Input: part model. Units: mm. Frame: model coordinates. Face numbers are marked on the shaded views. A direction names the side the tool comes from. Coordinates: 2 decimals unless noted, no trailing zeros. Loops run counter-clockwise (first coordinate to the right, second up) from the corner with the lowest first, then second, coordinate; pieces in that order, holes last. Notation, with made-up numbers: (9, -18.75) - (17, -18.75) arc R29 ccw to (17, 19.25) - close; hole circle Ø2 at (58.5, 2). An arc over 180 degrees is marked (long way). Use one line per item in the form item = value.
Autodesk Fusion 360 part; units mm, degrees
sketch "Back plate disc" plane through (0, 0, 0) normal (0, 0, 1) x (1, 0, 0)
  circle A0 centre (0, 0) radius 49
  dimension "d21" = 98
extrude "Main body extrude" add sketch "Back plate disc" along normal blind 23.2
sketch "Motor top outer ring sketch" plane through (0, 0, 23.2) normal (0, 0, 1) x (-1, 0, 0)
  circle A0 centre (0, 0) radius 49
  circle A1 centre (0, 0) radius 24
  dimension "d24" = 48
extrude "Motor top, outer ring extrude" add sketch "Motor top outer ring sketch" along normal blind 1.3 contours A1
sketch "Motor rotor ring sketch" plane through (0, 0, 24.5) normal (0, 0, 1) x (-1, 0, 0)
  circle A0 centre (0, 0) radius 24
  circle A1 centre (0, 0) radius 18.5
  dimension "d27" = 37
extrude "Motor rotor ring extrude" add sketch "Motor rotor ring sketch" along normal blind 1.7 contours A1
sketch "Motor driver cavity" plane through (0, 0, 0) normal (0, 0, 1) x (1, 0, 0)
  line L0 (-20.3145, 29.1131) -> (20.3145, 29.1131)
  arc A0 (-20.3145, 29.1131) -> (20.3145, 29.1131) centre (0, 0) ccw
  dimension "d30" = 71
extrude "Motor driver cavity extrude" add sketch "Motor driver cavity" against normal blind 11
sketch "Back plate mounting screws" plane through (0, 0, 0) normal (0, 0, -1) x (1, 0, 0)
  circle A0 centre (0, 0) radius 49
  circle A1 centre (0, 0) radius 42.5 construction
  circle A2 centre (16.1961, 39.293) radius 1.7
  circle A3 centre (-16.332, 39.2367) radius 1.7
  circle A4 centre (-39.293, 16.1961) radius 1.7
  circle A5 centre (-39.2367, -16.332) radius 1.7
  circle A6 centre (-16.1961, -39.293) radius 1.7
  circle A7 centre (16.332, -39.2367) radius 1.7
  circle A8 centre (39.293, -16.1961) radius 1.7
  circle A9 centre (39.2367, 16.332) radius 1.7
  line L0 (20.3145, -29.1131) -> (-20.3145, -29.1131)
  arc A10 (20.3145, -29.1131) -> (-20.3145, -29.1131) centre (0, 0) ccw
  dimension "d33" = 85
  dimension "d35" = 3.4
  dimension "d37" = 360
extrude "Representative M3 screw holes" cut sketch "Back plate mounting screws" against normal blind 2.5 contours A2 | A3 | A4 | A5 | A6 | A7 | A8 | A9
sketch "Top plate outer screw holes" plane through (0, 0, 23.2) normal (0, 0, 1) x (-1, 0, 0)
  circle A0 centre (0, 0) radius 24
  circle A1 centre (0, 0) radius 49
  circle A2 centre (0, 0) radius 42.5 construction
  circle A3 centre (-16.267, -39.2723) radius 1.7
  circle A4 centre (16.2672, -39.2722) radius 1.7
  circle A5 centre (39.2723, -16.267) radius 1.7
  circle A6 centre (39.2722, 16.2672) radius 1.7
  circle A7 centre (16.267, 39.2723) radius 1.7
  circle A8 centre (-16.2672, 39.2722) radius 1.7
  circle A9 centre (-39.2723, 16.267) radius 1.7
  circle A10 centre (-39.2722, -16.2672) radius 1.7
  dimension "d38" = 85
  dimension "d40" = 3.4
  dimension "d42" = 360
extrude "Representative screw extrudes" cut sketch "Top plate outer screw holes" against normal blind 2.5 contours A3 | A4 | A5 | A6 | A7 | A8 | A9 | A10
sketch "Motor shaft screws" plane through (0, 0, 26.2) normal (0, 0, 1) x (-1, 0, 0)
  circle A0 centre (0, 0) radius 18.5
  circle A1 centre (0, 0) radius 14 construction
  circle A2 centre (-6.9901, -12.13) radius 2.2
  dimension "d56" = 28
  dimension "d58" = 4.4
extrude "Motor shaft M4 screw extrude" cut sketch "Motor shaft screws" against normal blind 3.5 contours A2
pattern_circular "6 screws for rotor" count 6 over 360 about axis through (0, 0, 1.75) along (0, 0, 1) of "Motor shaft M4 screw extrude"
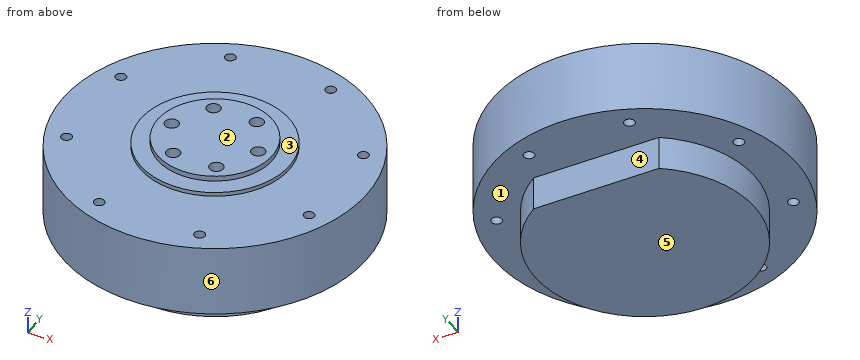
Q1. Cut plane C-C, the plane z = 7. Return loops of the section in (x, y).
Check values:
outline = circle Ø98 at (0, 0)
Q2. Cut plane A-A, the plane y = 27. Return loops of the section in (x, z), then the cut area to 3 significant figures.
Check values:
outline = (-40.89, 0) - (-23.05, 0) - (-23.05, -11) - (23.05, -11) - (23.05, 0) - (40.89, 0) - (40.89, 23.2) - (-40.89, 23.2) - close
area = 2,400 mm²
Q3. Set-up query: the marked faces 1, 2, 3 and 4. Return all of +Z, -Z, +X, -X, +Y, -Y with unobstructed straight access to the full face (end or side cutting, diameter ignored); none if empty.
Check values:
face_1 = -Z
face_2 = +Z, +X, -X, +Y, -Y
face_3 = +Z
face_4 = -Z, +X, -X, +Y
Q4. First-contact query: P1, Ø4, axis at x = 17, z = 18.5, coming from the -Y side; P2, Ø1.7, axis at x = 39, y = -16, coming from the -Z side; P3, Ø5, axis at x = 9.5, z = 18, coming from the -Y side. Flat tips, straight axial feed; report the tip coordinate or a pass-through.
Check values:
P1 = -46.65
P2 = 2.5
P3 = -48.5
Q5. Pull-direction query (X, two-part tool) for the marked faces 5 and 6; classes: pulls with the +X half, pulls with the -X half, needs draft (parallel to the pull), parting line crosses it, or undercut.
Check values:
face_5 = needs draft
face_6 = parting line crosses it
Q6. Ray query, line 1 along Z through (x, y) = (14.5, -18.5); line 2 along Z through (x, y) = (-19, -19); line 3 along X through (y, z) = (12.13, 25.3). Return the intervals inside material, ascending. Write a range as [from, to].
Check values:
line_1 = [-11, 24.5]
line_2 = [-11, 23.2]
line_3 = [-13.97, -9.21], [-4.81, 4.79], [9.19, 13.97]
Q7. Cut plane D-D, the plane y = -6. Return loops of the section in (x, z), then the cut area to 3 significant figures.
Check values:
outline = (-48.63, 0) - (-34.99, 0) - (-34.99, -11) - (34.99, -11) - (34.99, 0) - (48.63, 0) - (48.63, 23.2) - (23.24, 23.2) - (23.24, 24.5) - (17.5, 24.5) - (17.5, 26.2) - (-17.5, 26.2) - (-17.5, 24.5) - (-23.24, 24.5) - (-23.24, 23.2) - (-48.63, 23.2) - close
area = 3,150 mm²
Q8. Cut plane B-B, the plane x = -3. Return loops of the section in (y, z), then the cut area to 3 significant figures.
Check values:
outline = (-48.91, 0) - (-35.37, 0) - (-35.37, -11) - (29.11, -11) - (29.11, 0) - (48.91, 0) - (48.91, 23.2) - (23.81, 23.2) - (23.81, 24.5) - (18.26, 24.5) - (18.26, 26.2) - (-18.26, 26.2) - (-18.26, 24.5) - (-23.81, 24.5) - (-23.81, 23.2) - (-48.91, 23.2) - close
area = 3,100 mm²
